```python
from build123d import *

# Parameters (mm, degrees)
MID_CLIP_DEPTH              = 4
REAR_CLIP_DEPTH             = 4
SZKIC4_W                    = 43.5
SZKIC4_H                    = 64
DODANIE_WYCI_GNI_CIE3_DEPTH = 8


with BuildPart() as part:
    # Szkic2 → Mid Clip (new, symmetric)
    with BuildSketch(Plane(origin=(0, -36, 0), x_dir=(1, 0, 0), z_dir=(0, 1, 0))):
        with BuildLine():
            Line((52, 8), (0, 8))
            Line((0, 8), (0, -4))
            Line((0, -4), (47.9, -4))
            Line((47.9, -4), (47.9, 0))
            ThreePointArc((47.9, 0), (53.501665742, 3.815101571), (55, -2.794637722))
            Line((55, -2.794637722), (57.853658537, -5.452951654))
            ThreePointArc((57.853658537, -5.452951654), (59.335653114, 3.191894952), (52, 8))
        make_face()
    mid_clip = extrude(amount=MID_CLIP_DEPTH, both=True)



with BuildPart() as body_2:
    # Szkic3 → Rear Clip (new, symmetric)
    with BuildSketch(Plane(origin=(0, 36, 0), x_dir=(1, 0, 0), z_dir=(0, 1, 0))):
        with BuildLine():
            Line((53, 8), (0, 8))
            Line((0, 8), (0, -4))
            Line((0, -4), (48.9, -4))
            Line((48.9, -4), (48.9, 0))
            ThreePointArc((48.9, 0), (54.501665742, 3.815101571), (56, -2.794637722))
            Line((56, -2.794637722), (58.853658537, -5.452951654))
            ThreePointArc((58.853658537, -5.452951654), (60.335653114, 3.191894952), (53, 8))
        make_face()
    rear_clip = extrude(amount=REAR_CLIP_DEPTH, both=True)


with BuildPart() as part_1:
    add(part.part)

    add(body_2.part)  # Dodanie-wyci_gni_cie3 merges body 2
    # Szkic4 → Dodanie-wyci_gni_cie3 (add)
    with BuildSketch(Plane(origin=(0, 0, -8), x_dir=(-1, 0, 0), z_dir=(0, 0, -1))):
        with Locations((-21.75, 0)):
            Rectangle(SZKIC4_W, SZKIC4_H)
    dodanie_wyci_gni_cie3 = extrude(amount=-DODANIE_WYCI_GNI_CIE3_DEPTH)

    # Lustro2: Mid Clip, Rear Clip, Dodanie-wyci_gni_cie3 across plane
    add(mid_clip.mirror(Plane(origin=(0, -40, -8), x_dir=(0, 0, 1), z_dir=(-1, 0, 0))))
    add(rear_clip.mirror(Plane(origin=(0, -40, -8), x_dir=(0, 0, 1), z_dir=(-1, 0, 0))))
    add(dodanie_wyci_gni_cie3.mirror(Plane(origin=(0, -40, -8), x_dir=(0, 0, 1), z_dir=(-1, 0, 0))))


solid = part_1.part
```
The model under review builds one solid part; all positions refer to its coordinate system, in mm. A direction names the side the tool comes from. Round coordinates to 2 decimals unless told otherwise and drop trailing zeros. Order: outer loops, then holes, each group sorted by start corner. A loop starts at its lowest first (then second) coordinate and runs counter-clockwise, first axis right, second up.
(1) Mouldability with a two-part tool opening along Y and no side actions: class faces 6 (the face through (1, 36, 4)), 7 (the face through (0, -32, 1)) as released by +Y, released by -Y, zero draft, split by the parting line, or undercut.
Working result:
face 6: zero draft
face 7: undercut
(2) Take a section at C-C, the plane z = -2. State the section outline as (x, y) points.
Working result:
outline: (-60.75, 32) - (-56.58, 32) - (-56.58, 40) - (-60.75, 40) - close; (-59.75, -40) - (-55.58, -40) - (-55.58, -32) - (-59.75, -32) - close; (-49.42, 32) - (-43.5, 32) - (-43.5, -32) - (-48.42, -32) - (-48.42, -40) - (48.42, -40) - (48.42, -32) - (43.5, -32) - (43.5, 32) - (49.42, 32) - (49.42, 40) - (-49.42, 40) - close; (55.58, -40) - (59.75, -40) - (59.75, -32) - (55.58, -32) - close; (56.58, 32) - (60.75, 32) - (60.75, 40) - (56.58, 40) - close
(3) Take a section at D-D, the plane y = -20.5. State the section outline as (x, z) points, plus the area to 3 significant figures.
Working result:
outline: (-43.5, -8) - (43.5, -8) - (43.5, 0) - (-43.5, 0) - close
area: 696 mm2
(4) Take a section at B-B, the plane x = -33.5. State the section outline as (y, z) points.
Working result:
outline: (-40, -8) - (40, -8) - (40, 4) - (32, 4) - (32, 0) - (-32, 0) - (-32, 4) - (-40, 4) - close
(5) Tool access review of faces 1 (the face through (48.9, 36, 2)), 2 (the face through (-1, 0, 0)), 3 (the face through (0, 32, 1)), 4 (the face through (-57.4, 36.1, 4.1)), 5 (the face through (-47.9, -36, 2)): name each direction out of +Z, -Z, +X, -X, +Y, -Y from which nothing blocks a thin tool from reaching the whole face with its end or side.
Working result:
face 1: +Z, +Y, -Y
face 2: +Z, +X, -X
face 3: +Z
face 4: +Z, +Y
face 5: +Z, -Y
(6) Take a section at A-A, the plane y = -35. State the section outline as (x, z) points, plus the area to 3 significant figures.
Working result:
outline: (-57.85, 5.45) arc R8 ccw to (-52, -8) - (52, -8) arc R8 ccw to (57.85, 5.45) - (55, 2.79) arc R4.1 cw (long way) to (47.9, 0) - (47.9, 4) - (-47.9, 4) - (-47.9, 0) arc R4.1 cw (long way) to (-55, 2.79) - close
area: 1,300 mm2
(7) For P1, Ø2, axis at y = 34.5, z = 2, coming from the -X side; P2, Ø8, axis at x = -44, y = -16.5, coming from the -Z side; P3, Ø4, axis at y = 3.5, z = -6, coming from the -X side; P4, Ø7.5, axis at x = 52, z = 0, coming from the -Y side, all flat-tipped, find the tip position at first contact; note any pin that passes through.
Working result:
P1: stops at x = -60.94
P2: stops at z = -8
P3: stops at x = -43.5
P4: stops at y = 32
(8) Wall thickness on L1, parallel to X at y = -38.5, z = 0; L2, parallel to X at y = 38.25, z = 0; L3, parallel to Y at x = 51, z = -7: over which ranges is each line inside the solid? List them lowest first.
Working result:
L1: x = -60 to -56.1, -47.9 to 47.9, 56.1 to 60
L2: x = -61 to -57.1, -48.9 to 48.9, 57.1 to 61
L3: y = -40 to -32, 32 to 40
